CAD build for the part. Positions are in the model's coordinates, mm. A direction names the side the tool comes from. Round coordinates to 2 decimals unless told otherwise and drop trailing zeros. Loops run counter-clockwise (first coordinate to the right, second up) from the corner with the lowest first, then second, coordinate; pieces in that order, holes last.
```python
from build123d import *

# Parameters (mm, degrees)
PAD_DEPTH    = 40
SKETCH001_W  = 12
SKETCH001_H  = 10
SKETCH001_R  = 1.6
PAD001_DEPTH = 2
SKETCH002_R  = 1.55
PAD002_DEPTH = 2
POCKET_DEPTH = 5


with BuildPart() as part:
    # Sketch → Pad (new body)
    with BuildSketch(Plane.YZ):
        with BuildLine():
            Line((-5, 8), (-5, 9))
            Line((-5, 9), (-6, 9))
            Line((-6, 9), (-6, -1))
            Line((-6, -1), (6, -1))
            Line((6, -1), (6, 9))
            Line((6, 9), (5, 9))
            Line((5, 9), (5, 8))
            ThreePointArc((5, 8), (3.556624, 5.5), (5, 3))
            Line((5, 3), (5, 0))
            Line((5, 0), (2.5, 0))
            ThreePointArc((2.5, 0), (0, 1.443376), (-2.5, 0))
            Line((-2.5, 0), (-5, 0))
            Line((-5, 0), (-5, 3))
            ThreePointArc((-5, 3), (-3.556624, 5.5), (-5, 8))
        make_face()
    extrude(amount=PAD_DEPTH)

    # Sketch001 (on Face15 of Pad) → Pad001 (join)
    with BuildSketch(Plane(origin=(0, 0, 0), x_dir=(0, 1, 0), z_dir=(-1, 0, 0))):
        with Locations((0, -4)):
            Rectangle(SKETCH001_W, SKETCH001_H)
        with Locations((0, -5)):
            Circle(SKETCH001_R, mode=Mode.SUBTRACT)
    extrude(amount=PAD001_DEPTH)

    # Sketch002 (on Face5 of Pad001) → Pad002 (join)
    with BuildSketch(Plane.YZ.offset(40)):
        with BuildLine():
            ThreePointArc((-6, 9), (-10, 13), (-14, 9))
            Line((-14, 9), (-14, -1))
            ThreePointArc((-14, -1), (-12.828427, -3.828427), (-10, -5))
            Line((10, -5), (-10, -5))
            ThreePointArc((10, -5), (12.828427, -3.828427), (14, -1))
            Line((14, 9), (14, -1))
            ThreePointArc((14, 9), (10, 13), (6, 9))
            Line((5, 0), (6, 9))
            Line((-5, 0), (5, 0))
            Line((-6, 9), (-5, 0))
        make_face()
        with Locations((-10, 9)):
            Circle(SKETCH002_R, mode=Mode.SUBTRACT)
        with Locations((10, 9)):
            Circle(SKETCH002_R, mode=Mode.SUBTRACT)
        with Locations((10, -1)):
            Circle(SKETCH002_R, mode=Mode.SUBTRACT)
        with Locations((-10, -1)):
            Circle(SKETCH002_R, mode=Mode.SUBTRACT)
    extrude(amount=-PAD002_DEPTH)

    # Sketch003 (on Face7 of Pad002) → Pocket (cut)
    with BuildSketch(Plane(origin=(0, -6, 0), x_dir=(0, 0, -1), z_dir=(0, -1, 0))):
        with BuildLine():
            Line((-9, 0.4), (-4.5, 0.4))
            ThreePointArc((-4.5, 0.4), (-3.085786, 0.985786), (-2.5, 2.4))
            Line((-2.5, 2.4), (-2.5, 5.4))
            Line((-2.5, 5.4), (-9, 5.4))
            Line((-9, 5.4), (-9, 0.4))
        make_face()
    extrude(amount=-POCKET_DEPTH, mode=Mode.SUBTRACT)


solid = part.part
```
Item 1: Cut at A-A, the plane y = -0.75. Give the cut face in (x, z).
Answers follow:
outline: (-2, -1) - (38, -1) - (38, -5) - (40, -5) - (40, 1.34) - (0, 1.34) - (0, 3.59) - (-2, 3.59) - close; (-2, 6.41) - (0, 6.41) - (0, 9) - (-2, 9) - close
Item 2: Two-plate mould, pull along Z, no slides. Class faces 1 (the flat face through (3.9, -5.5, 2.5)), 2 (the cylindrical face through (39.01, -11.23, 8.06)), 3 (the flat face through (22.5, -5, 8.5)): released by +Z, released by -Z, zero draft, split by the parting line, or undercut.
Answers follow:
face 1: released by +Z
face 2: undercut
face 3: zero draft
Item 3: Cut at B-B, the plane z = 5. Give the cut face in (x, y), plus the area to 3 significant figures.
Answers follow:
outline: (-2, -6) - (0.4, -6) - (0.4, -3.6) - (0, -3.6) - (0, -1.6) - (-2, -1.6) - close; (-2, 1.6) - (0, 1.6) - (0, 3.6) - (40, 3.6) - (40, 14) - (38, 14) - (38, 6) - (-2, 6) - close; (5.4, -6) - (38, -6) - (38, -14) - (40, -14) - (40, -3.6) - (5.4, -3.6) - close
area: 230 mm2
Item 4: Probe line 1 (Z direction, x = 38.95, y = -10); line 2 (Z direction, x = -1.5, y = 0); line 3 (Y direction, x = 25.5, z = 2). List the from-to ranges inside material, lowest first.
Answers follow:
line 1: z = -5 to -2.55, 0.55 to 7.45, 10.55 to 13
line 2: z = -1 to 3.4, 6.6 to 9
line 3: y = -6 to -5, 5 to 6
Item 5: Cut at C-C, the plane x = 27.5. Give the cut face in (y, z).
Answers follow:
outline: (-6, -1) - (6, -1) - (6, 9) - (5, 9) - (5, 8) arc R2.89 ccw to (5, 3) - (5, 0) - (2.5, 0) arc R2.89 ccw to (-2.5, 0) - (-5, 0) - (-5, 3) arc R2.89 ccw to (-5, 8) - (-5, 9) - (-6, 9) - close
Item 6: Flat gauge pins, fed straight in: P1, Ø3.5, axis at y = 0, z = 5, coming from the +X side; P2, Ø4, axis at y = -9, z = -1.5, coming from the -X side; P3, Ø3, axis at x = 11, y = 2.5, coming from the +Z side; P4, Ø1.9, axis at y = 10, z = -1, coming from the +X side. Where does each tip first touch, or does it go through?
Answers follow:
P1: stops at x = 0
P2: stops at x = 38
P3: stops at z = 7.04
P4: passes through
Item 7: Cut at D-D, the plane z = 12. Give the cut face in (x, y).
Answers follow:
outline: (38, -12.65) - (40, -12.65) - (40, -7.35) - (38, -7.35) - close; (38, 7.35) - (40, 7.35) - (40, 12.65) - (38, 12.65) - close
Item 8: 3-axis set-ups, long thin cutter, end or side, ignore diameter. For faces 4 (the cylindrical face through (19.72, 0.042, 1.443)), 5 (the flat face through (18, 0, -1)), 6 (the flat face through (18, 6, 4)), 7 (the flat face through (0.4, -5, 6)): which of +Z, -Z, +X, -X, +Y, -Y reach the whole face in a straight line?
Answers follow:
face 4: +Z, +X
face 5: -Z, -X, +Y, -Y
face 6: +Z, -Z, -X, +Y
face 7: +Z, -Y
